Geometry: final body of the model. Coordinates: model frame, mm. Give positions to 0.01 mm unless a question says otherwise; leave off trailing zeros. Write each loop counter-clockwise with the first axis right and the second up, starting at its lowest first coordinate (ties: lowest second). Pieces come first, ordered by that corner, then holes.
```python
from build123d import *

# Parameters (mm, degrees)
BOSS_EXTRUDE1_DEPTH = 2.95
SKETCH5_R           = 3.3
HOLE1_DEPTH         = 81.293387804
SKETCH7_R           = 2.5
CUT_EXTRUDE2_DEPTH  = 81.293387804


with BuildPart() as part:
    # Sketch1 → Boss-Extrude1 (new body)
    with BuildSketch(Plane(origin=(0, 0, 0), x_dir=(1, 0, 0), z_dir=(0, 1, 0))):
        with BuildLine():
            Line((-44.475, 0), (44.475, 0))
            ThreePointArc((44.475, 0), (53.243124087, 3.631875913), (56.875, 12.4))
            Line((56.875, 12.4), (56.875, 56.6))
            Line((56.875, 56.6), (-56.875, 56.6))
            Line((-56.875, 56.6), (-56.875, 12.4))
            ThreePointArc((-56.875, 12.4), (-53.243124087, 3.631875913), (-44.475, 0))
        make_face()
    extrude(amount=BOSS_EXTRUDE1_DEPTH)

    # Sketch5 → Hole1 (cut, through all)
    with BuildSketch(Plane(origin=(0, 2.95, 0), x_dir=(1, 0, 0), z_dir=(0, 1, 0))):
        with Locations(Location((-41, 25.2, 0), (0, 0, 270))):
            Circle(SKETCH5_R)
        with Locations(Location((-24.6, 25.2, 0), (0, 0, 270))):
            Circle(SKETCH5_R)
        with Locations(Location((-8.2, 25.2, 0), (0, 0, 270))):
            Circle(SKETCH5_R)
        with Locations(Location((8.2, 25.2, 0), (0, 0, 270))):
            Circle(SKETCH5_R)
        with Locations(Location((24.6, 25.2, 0), (0, 0, 270))):
            Circle(SKETCH5_R)
        with Locations(Location((41, 25.2, 0), (0, 0, 270))):
            Circle(SKETCH5_R)
    extrude(amount=-HOLE1_DEPTH, mode=Mode.SUBTRACT)

    # Sketch7 → Cut-Extrude2 (cut, through all)
    with BuildSketch(Plane(origin=(0, 2.95, 0), x_dir=(1, 0, 0), z_dir=(0, 1, 0))):
        with Locations(Location((-37.975, 44.2, 0), (0, 0, 270))):
            Circle(SKETCH7_R)
    cut_extrude2 = extrude(amount=-CUT_EXTRUDE2_DEPTH, mode=Mode.SUBTRACT)

    # Mirror1: Cut-Extrude2 across plane
    add(cut_extrude2.mirror(Plane(origin=(0, 0, 0), x_dir=(0, 0, 1), z_dir=(1, 0, 0))), mode=Mode.SUBTRACT)


solid = part.part
```
Item 1: Pin query (flat end, axial travel): pin 1 Ø4 at (x, z) = (37.975, -44.2) entering from +Y. Return the tip coordinate at first contact, or that it passes through.
Found:
pin 1: passes through
Item 2: Pull-direction query (Z, two-part tool) for faces 1 (the face through (-56.875, 1, -35)), 2 (the face through (1, 1, -56.6)), 3 (the face through (43.23, 1.5, -27.63)); classes: +Z half, -Z half, draft (parallel to the pull), parting line (faces both ways), or undercut.
Found:
face 1: draft
face 2: -Z half
face 3: undercut
Item 3: Section C-C, the plane y = 2.3. State how many separate pieces and enclosed holes the cut face has, plus the area to 3 significant figures.
Found:
separate pieces: 1
enclosed holes: 8
area: 6,130 mm2
Item 4: Line query: L1, parallel to X at y = 0.95, z = -44.2 (3 decimals); L2, parallel to Z at x = -26, y = 1.7; L3, parallel to X at y = 2.75, z = -45.5 (3 decimals). Output: solid intervals per line, ascending.
Found:
L1: x = -56.875 to -40.475, -35.475 to 35.475, 40.475 to 56.875
L2: z = -56.6 to -28.19, -22.21 to 0
L3: x = -56.875 to -40.11, -35.84 to 35.84, 40.11 to 56.875
Item 5: Section B-B, the plane z = -25.2. Return the cut outline in (x, y) (3 decimals), plus the area to 3 significant figures.
Found:
outline: (-56.875, 0) - (-44.3, 0) - (-44.3, 2.95) - (-56.875, 2.95) - close; (-37.7, 0) - (-27.9, 0) - (-27.9, 2.95) - (-37.7, 2.95) - close; (-21.3, 0) - (-11.5, 0) - (-11.5, 2.95) - (-21.3, 2.95) - close; (-4.9, 0) - (4.9, 0) - (4.9, 2.95) - (-4.9, 2.95) - close; (11.5, 0) - (21.3, 0) - (21.3, 2.95) - (11.5, 2.95) - close; (27.9, 0) - (37.7, 0) - (37.7, 2.95) - (27.9, 2.95) - close; (44.3, 0) - (56.875, 0) - (56.875, 2.95) - (44.3, 2.95) - close
area: 219 mm2
Item 6: Section D-D, the plane z = -43. Return the cut outline in (x, y) (3 decimals), plus the area to 3 significant figures.
Found:
outline: (-56.875, 0) - (-40.168, 0) - (-40.168, 2.95) - (-56.875, 2.95) - close; (-35.782, 0) - (35.782, 0) - (35.782, 2.95) - (-35.782, 2.95) - close; (40.168, 0) - (56.875, 0) - (56.875, 2.95) - (40.168, 2.95) - close
area: 310 mm2
Item 7: Section A-A, the plane x = 24.6. Return the cut outline in (y, z), plus the area to 4 significant figures.
Found:
outline: (0, -56.6) - (2.95, -56.6) - (2.95, -28.5) - (0, -28.5) - close; (0, -21.9) - (2.95, -21.9) - (2.95, 0) - (0, 0) - close
area: 147.5 mm2
